Geometry: see drawing. Coordinates: mm, zero at the bounding-box minimum. A direction names the side the tool comes from. Round coordinates to 2 decimals unless told otherwise and drop trailing zeros. Loops run counter-clockwise (first coordinate to the right, second up) from the corner with the lowest first, then second, coordinate; pieces in that order, holes last.
(1) First-contact query: pin 1 Ø5 at (x, y) = (20.5, 27.5) entering from +Z; pin 2 Ø2.5 at (x, y) = (10, 12) entering from +Z; pin 3 Ø3 at (x, y) = (11.5, 17.5) entering from +Z; pin 4 Ø2 at (x, z) = (22.5, 10) entering from -Y. Flat tips, straight axial feed; report the tip coordinate or a pass-through.
(2) Section B-B, the plane x = 10.5. Return the cut outline in (y, z), plus the area to 3 significant figures.
(3) Material intervals for probe 1 along Y at (x, z) = (10, 4.15); probe 2 along X at (y, z) = (12, 4.5); probe 3 along Y at (x, z) = (10, 1.55), sorted ascending.
(4) Mould query, pull axis Y, two halves, no side actions, for the marked faces 1, 2, 3 and 4. Classes: pulls with the +Y half, pulls with the -Y half, needs draft (parallel to the pull), parting line crosses it, or undercut.
(5) Section C-C, the plane y = 29. Return the cut outline in (x, z).
(6) Section D-D, the plane x = 15.5. Return the cut outline in (y, z).
(7) Section A-A, the plane y = 24. Return the cut outline in (x, z), plus the area to 4 significant figures.
(8) Set-up query: the marked faces 5, 6 and 7. Return all of +Z, -Z, +X, -X, +Y, -Y with unobstructed straight access to the full face (end or side cutting, diameter ignored); none if empty.
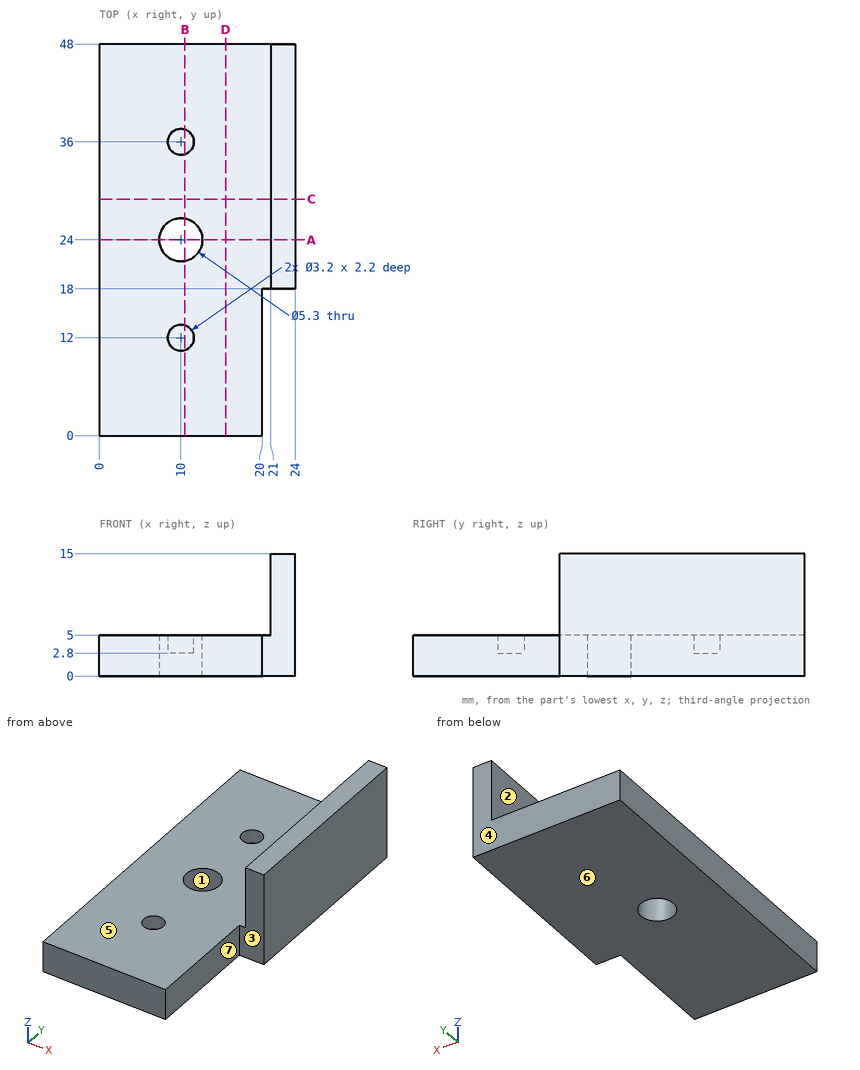
Output values:
1. pin 1: stops at z = 15
1. pin 2: stops at z = 2.8
1. pin 3: stops at z = 5
1. pin 4: stops at y = 18
2. outline: (0, 0) - (21.4, 0) - (21.4, 5) - (13.52, 5) - (13.52, 2.8) - (10.48, 2.8) - (10.48, 5) - (0, 5) - close; (26.6, 0) - (48, 0) - (48, 5) - (37.52, 5) - (37.52, 2.8) - (34.48, 2.8) - (34.48, 5) - (26.6, 5) - close
2. area: 201 mm2
3. probe 1: y = 0 to 10.4, 13.6 to 21.35, 26.65 to 34.4, 37.6 to 48
3. probe 2: x = 0 to 8.4, 11.6 to 20
3. probe 3: y = 0 to 21.35, 26.65 to 48
4. face 1: undercut
4. face 2: needs draft
4. face 3: pulls with the -Y half
4. face 4: pulls with the +Y half
5. outline: (0, 0) - (24, 0) - (24, 15) - (21, 15) - (21, 5) - (0, 5) - close
6. outline: (0, 0) - (48, 0) - (48, 5) - (0, 5) - close
7. outline: (0, 0) - (7.35, 0) - (7.35, 5) - (0, 5) - close; (12.65, 0) - (24, 0) - (24, 15) - (21, 15) - (21, 5) - (12.65, 5) - close
7. area: 123.5 mm2
8. face 5: +Z, -X, +Y, -Y
8. face 6: -Z, +X, -X, +Y, -Y
8. face 7: +Z, -Z, +X, -Y
